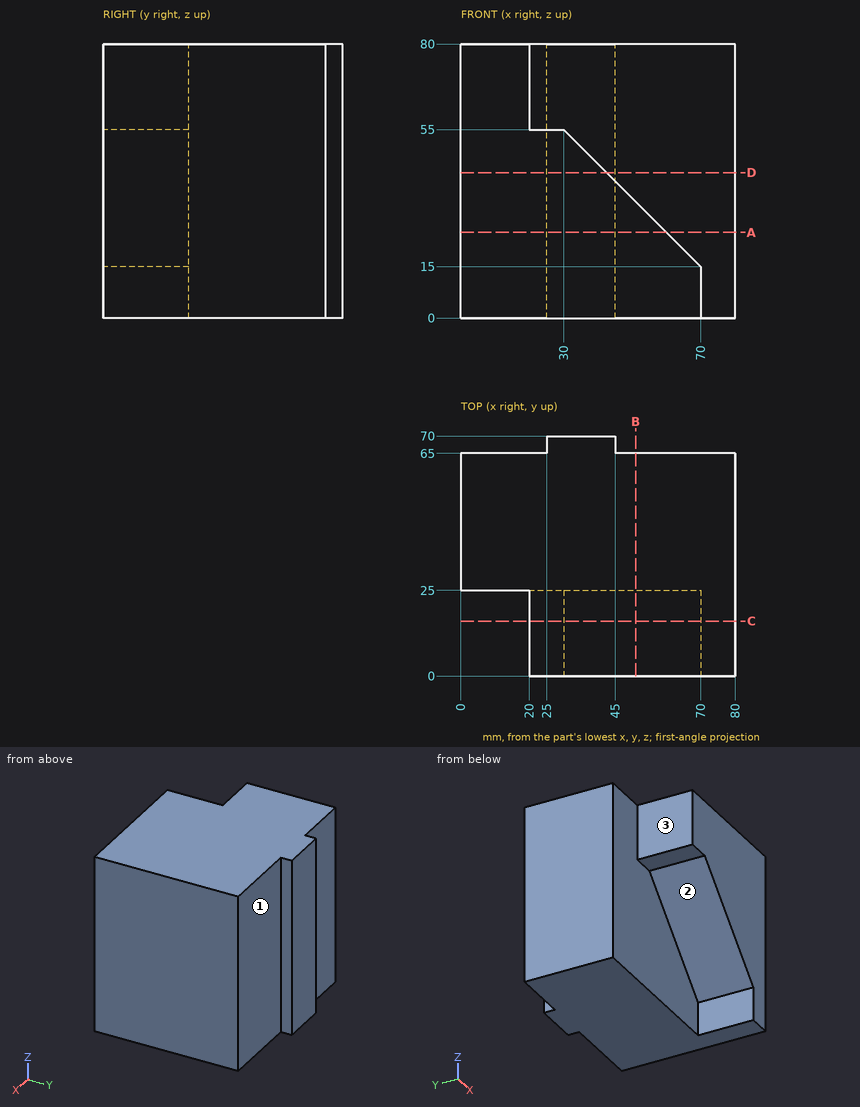
Geometry check sheet. Reference: drawing and pictorial views, mm from the part's lowest x, y, z. A direction names the side the tool comes from. Coordinates: 2 decimals unless noted, no trailing zeros. Order: outer loops, then holes, each group sorted by start corner. A loop starts at its lowest first (then second) coordinate and runs counter-clockwise, first axis right, second up. Notation, with made-up numbers: (-4, 61.5) -> (36, 61.5) arc R30 ccw to (36, 91.5) -> close; hole circle Ø10 at (-33, 17.25). An arc over 180 degrees is marked (long way). Write item = value, one per line. Start each with the question number.
1) Access from +Z, -Z, +X, -X, +Y, -Y to the whole of each face (thin tool, end or side, straight path). Record for the marked faces 1, 2 and 3.
2) Cross-section at C-C (y = 16). Enter the section's corners in (x, z).
3) Cross-section at A-A (z = 25). Enter the section's corners in (x, y).
4) Cross-section at D-D (z = 42.5). Enter the section's corners in (x, y), then the cut area to 3 significant figures.
5) Go/stop test with flat-tipped pins: P1, Ø7.5, axis at y = 11.5, z = 63.5, coming from the -X side; P2, Ø12, axis at y = 14.5, z = 7.5, coming from the -X side; P3, Ø4, axis at y = 67.5, z = 57, coming from the -X side. Record where each tip stops, or that it passes through.
6) Material ranges on L1, parallel to Y at x = 37, z = 46.5; L2, parallel to X at y = 15, z = 62; L3, parallel to X at y = 66.5, z = 72.5, recorded low to high.
7) Cross-section at B-B (x = 51). Enter the section's corners in (y, z), then the cut area to 3 significant figures.
Ans:
q1.face_1 = +Z, -Z, +X, +Y
q1.face_2 = -Z, -X, -Y
q1.face_3 = +Z, -Z, -X, -Y
q2.outline = (20, 55) -> (30, 55) -> (70, 15) -> (70, 0) -> (80, 0) -> (80, 80) -> (20, 80) -> close
q3.outline = (0, 25) -> (60, 25) -> (60, 0) -> (80, 0) -> (80, 65) -> (45, 65) -> (45, 70) -> (25, 70) -> (25, 65) -> (0, 65) -> close
q4.outline = (0, 25) -> (42.5, 25) -> (42.5, 0) -> (80, 0) -> (80, 65) -> (45, 65) -> (45, 70) -> (25, 70) -> (25, 65) -> (0, 65) -> close
q4.area = 4,240 mm²
q5.P1 = 20
q5.P2 = 70
q5.P3 = 25
q6.L1 = 25 to 70
q6.L2 = 20 to 80
q6.L3 = 25 to 45
q7.outline = (0, 34) -> (25, 34) -> (25, 0) -> (65, 0) -> (65, 80) -> (0, 80) -> close
q7.area = 4,350 mm²
